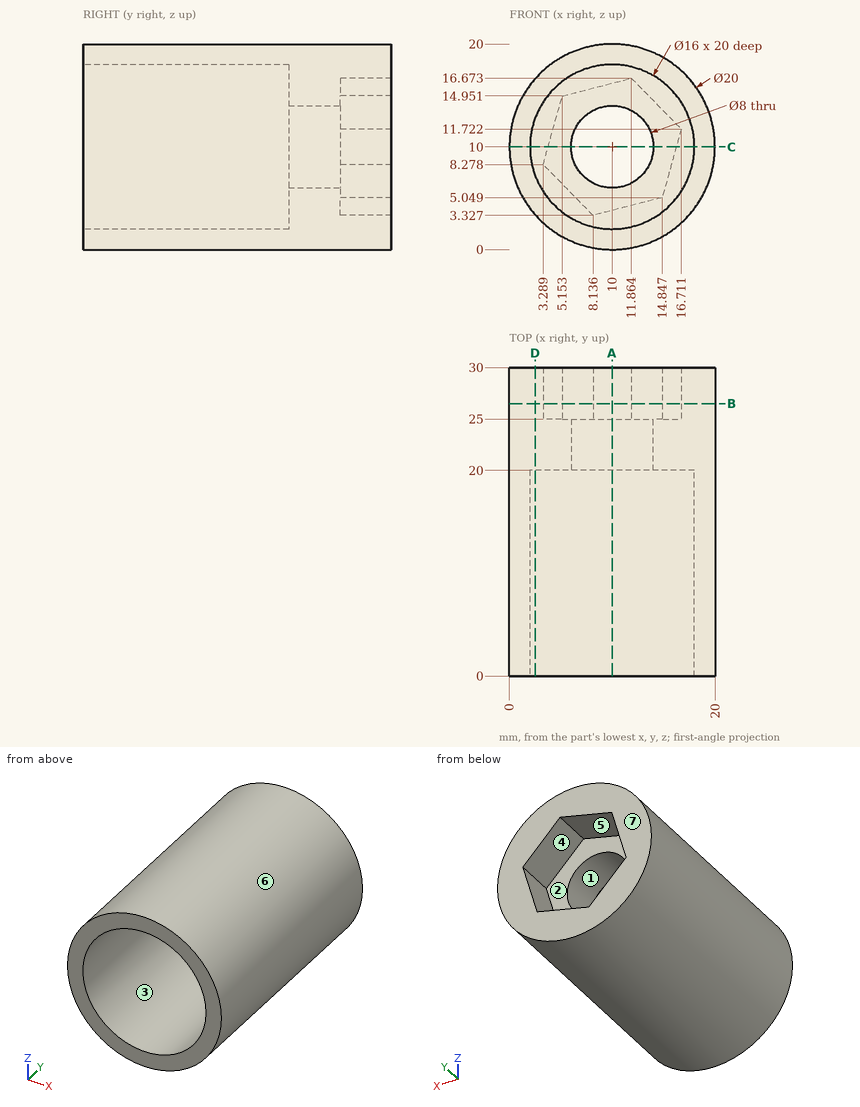
Geometry check sheet. Reference: drawing and pictorial views, mm from the part's lowest x, y, z. A direction names the side the tool comes from. Round coordinates to 2 decimals unless told otherwise and drop trailing zeros. Loops run counter-clockwise (first coordinate to the right, second up) from the corner with the lowest first, then second, coordinate; pieces in that order, holes last. Notation, with made-up numbers: (30.5, -13) - (89.5, -13) arc R26 cw to (89.5, 6) - close; hole circle Ø8 at (-26.5, 14). An arc over 180 degrees is marked (long way). Write item = value, one per line. Start each with the question number.
Q1. Section check A-A (x = 10). Record the boundary of the cut face in (y, z) (1 decimal), plus the area to 3 significant figures.
Q2. Depth check by flat-ended pin: P1, Ø5, axis at y = 7.5, z = 3, coming from the -X side; P2, Ø1.5, axis at x = 12, y = 15.5, coming from the -Z side; P3, Ø10.5, axis at x = 10, z = 10, coming from the +Y side; P4, Ø10, axis at y = 17.5, z = 7, coming from the -X side. Enter the tip coordinate at first touch or a pass-through.
Q3. Access from +Z, -Z, +X, -X, +Y, -Y to the whole of each face (thin tool, end or side, straight path). Record for the marked faces 1, 2 and 3.
Q4. Section check C-C (z = 10). Record the boundary of the cut face in (x, y), plus the area to 3 significant figures.
Q5. Release check for a two-part mould opening along X. For the marked faces 4, 5, 6 and 7 record: pulls with the +X half, pulls with the -X half, needs draft (parallel to the pull), parting line crosses it, or undercut.
Q6. Section check D-D (x = 2.5). Record the boundary of the cut face in (y, z) (1 decimal).
Q7. Thickness scan on L1, parallel to Z at x = 10, y = 21.6; L2, parallel to Z at x = 10, y = 6; L3, parallel to Y at x = 3, z = 12. Record the ranges inside material, lowest first.
Q8. Section check B-B (y = 26.5). Record the boundary of the cut face in (x, z).
Derived:
q1.outline = (0, 0) - (30, 0) - (30, 3.8) - (25, 3.8) - (25, 6) - (20, 6) - (20, 2) - (0, 2) - close; (0, 18) - (20, 18) - (20, 14) - (25, 14) - (25, 16.2) - (30, 16.2) - (30, 20) - (0, 20) - close
q1.area = 178 mm^2
q2.P1 = 1.07
q2.P2 = 0.08
q2.P3 = 25
q2.P4 = 0
q3.face_1 = +Y, -Y
q3.face_2 = +Y
q3.face_3 = -Y
q4.outline = (0, 0) - (2, 0) - (2, 20) - (6, 20) - (6, 25) - (3.77, 25) - (3.77, 30) - (0, 30) - close; (14, 20) - (18, 20) - (18, 0) - (20, 0) - (20, 30) - (16.23, 30) - (16.23, 25) - (14, 25) - close
q4.area = 178 mm^2
q5.face_4 = undercut
q5.face_5 = undercut
q5.face_6 = parting line crosses it
q5.face_7 = needs draft
q6.outline = (0, 3.4) - (30, 3.4) - (30, 16.6) - (0, 16.6) - (0, 12.8) - (20, 12.8) - (20, 7.2) - (0, 7.2) - close
q7.L1 = 0 to 6, 14 to 20
q7.L2 = 0 to 2, 18 to 20
q7.L3 = 20 to 30
q8.outline = circle Ø20 at (10, 10); hole (3.29, 8.28) - (8.14, 3.33) - (14.85, 5.05) - (16.71, 11.72) - (11.86, 16.67) - (5.15, 14.95) - close
